from build123d import *

# Parameters (mm, degrees)
SALIENTE_EXTRUIR1_DEPTH = 280
CROQUIS2_W              = 23
CROQUIS2_H              = 250
CORTAR_EXTRUIR1_DEPTH   = 3
CHAFL_N1_SIZE           = 10


with BuildPart() as part:
    # Croquis1 → Saliente-Extruir1 (new body)
    with BuildSketch(Plane(origin=(0, 0, 0), x_dir=(1, 0, 0), z_dir=(0, 1, 0))):
        Polygon((0, 0), (0, 38), (3, 38), (3, 3), (38, 3), (38, 0), align=None)
    extrude(amount=SALIENTE_EXTRUIR1_DEPTH)

    # Croquis2 → Cortar-Extruir1 (cut)
    with BuildSketch(Plane.ZY):
        with Locations((-26.5, 140)):
            Rectangle(CROQUIS2_W, CROQUIS2_H)
    extrude(amount=-CORTAR_EXTRUIR1_DEPTH, mode=Mode.SUBTRACT)

    # Chaflán1
    chafl_n1_edges = [part.edges().sort_by_distance(p)[0] for p in [
        (1.5, 265, -15),
        (1.5, 15, -15),
    ]]
    chamfer(chafl_n1_edges, length=CHAFL_N1_SIZE)


solid = part.part
Geometry check sheet. Reference: the model listing, model coordinates, mm. A direction names the side the tool comes from. Coordinates: 2 decimals unless noted, no trailing zeros. Order: outer loops, then holes, each group sorted by start corner. A loop starts at its lowest first (then second) coordinate and runs counter-clockwise, first axis right, second up. Notation, with made-up numbers: (63, 42.5) - (100, 42.5) arc R25 cw to (100, 79.5) - close; hole circle Ø1 at (38.25, -25). An arc over 180 degrees is marked (long way). Answer in a Markdown table with one row per item. Add a question column.
1) Cross-section at B-B, the plane y = 62. Record the cut outline in (x, z), then the cut area to 3 significant figures.
2) Release check for a two-part mould opening along Y. For faces 4 (the flat face through (11, 0, -2)), 5 (the flat face through (1, 260, -20)), 6 (the flat face through (0, 138, -10)) record: +Y half, -Y half, draft (parallel to the pull), parting line (faces both ways), or undercut.
3) Gauge pin test, flat ends, axial feed: P1, Ø17.5, axis at y = 94, z = -20, coming from the +X side; P2, Ø5, axis at x = 25.5, y = 178, coming from the -Z side; P3, Ø0.9, axis at x = 1.5, y = 184, coming from the -Z side. Record the tip position at first contact, or that the pin passes through.
4) Cross-section at A-A, the plane z = -29.5. Record the cut outline in (x, y), then the cut area to 3 significant figures.
5) Cross-section at D-D, the plane x = 11.5. Record the cut outline in (y, z).
6) Set-up check for faces 1 (the flat face through (20, 138, -3)), 2 (the flat face through (1, 20, -20)), 3 (the flat face through (11, 280, -2)): record each of +Z, -Z, +X, -X, +Y, -Y from which the full face is reachable in a straight line by a thin tool's end or side.
7) Cross-section at C-C, the plane z = -8. Record the cut outline in (x, y), then the cut area to 3 significant figures.
8) Material ranges on line 1 along Z through (x, y) = (22.5, 189.5); line 2 along X through (y, z) = (68.5, -14), recorded low to high. Write a range as [from, to].
Check result:
| question | item | result |
|---|---|---|
| 1 | outline | (0, -15) - (3, -15) - (3, -3) - (38, -3) - (38, 0) - (0, 0) - close |
| 1 | area | 150 mm² |
| 2 | face 4 | -Y half |
| 2 | face 5 | undercut |
| 2 | face 6 | draft |
| 3 | P1 | stops at x = 3 |
| 3 | P2 | stops at z = -3 |
| 3 | P3 | stops at z = -15 |
| 4 | outline | (0, 0) - (3, 0) - (3, 15) - (0, 15) - close; (0, 265) - (3, 265) - (3, 280) - (0, 280) - close |
| 4 | area | 90.0 mm² |
| 5 | outline | (0, -3) - (280, -3) - (280, 0) - (0, 0) - close |
| 6 | face 1 | -Z, +X, +Y, -Y |
| 6 | face 2 | -Z, +X, -X |
| 6 | face 3 | +Z, -Z, +X, -X, +Y |
| 7 | outline | (0, 0) - (3, 0) - (3, 280) - (0, 280) - close |
| 7 | area | 840 mm² |
| 8 | line 1 | z = [-3, 0] |
| 8 | line 2 | x = [0, 3] |
